```python
from build123d import *

# Parameters (mm, degrees)
SKETCH1_W           = 76.2
SKETCH1_H           = 76.2
SKETCH1_W_2         = 69.85
SKETCH1_H_2         = 69.85
EXTRUDE_THIN1_DEPTH = 38.1
SKETCH2_R           = 2.4892
CUT_EXTRUDE1_DEPTH  = 77.2


with BuildPart() as part:
    # Sketch1 → Extrude-Thin1 (new body, symmetric)
    with BuildSketch(Plane.XY):
        Rectangle(SKETCH1_W, SKETCH1_H)
        Rectangle(SKETCH1_W_2, SKETCH1_H_2, mode=Mode.SUBTRACT)
    extrude(amount=EXTRUDE_THIN1_DEPTH, both=True)

    # Sketch2 → Cut-Extrude1 (cut, through all)
    with BuildSketch(Plane.XZ.offset(38.1)):
        with Locations((0, 12.7)):
            Circle(SKETCH2_R)
        with Locations((0, -12.7)):
            Circle(SKETCH2_R)
    extrude(amount=-CUT_EXTRUDE1_DEPTH, mode=Mode.SUBTRACT)


solid = part.part
```
Here's how the part is built. I have some questions about the finished solid (model axes, mm). A direction names the side the tool comes from. Give positions to 0.01 mm unless a question says otherwise; leave off trailing zeros. Write each loop counter-clockwise with the first axis right and the second up, starting at its lowest first coordinate (ties: lowest second). Pieces come first, ordered by that corner, then holes. Notation, with made-up numbers: (62, -8) -> (107, -8) arc R25 cw to (107, 4) -> close; hole circle Ø6 at (4.5, 39). An arc over 180 degrees is marked (long way). Use one line per item in the form item = value.
1) I'm going to push a flat-ended pin straight in: pin 1 (4 mm diameter, centred on x = 0, z = 12.7, fed in from -Y). Where does the tip first touch, or does it pass through?
Verdict:
pin_1 = through
2) If I drill on L1, parallel to X at y = 20, z = -30.5 (3 decimals); L2, parallel to Z at x = 0, y = 35.7, over which ranges is the centre line in solid material (lowest first)? Write a range as [from, to].
Verdict:
L1 = [-38.1, -34.925], [34.925, 38.1]
L2 = [-38.1, -15.19], [-10.21, 10.21], [15.19, 38.1]
3) On a 3-axis mill with a long thin cutter (end or side, diameter ignored), from which of +Z, -Z, +X, -X, +Y, -Y can I reach the whole of each face in a straight line? I mean faces 4 (the face through (-3, -37, 38.1)), 5 (the face through (34.925, 0, 1)). Say none if no direction works.
Verdict:
face_4 = +Z, +X, -X, +Y, -Y
face_5 = +Z, -Z
4) Suppose I cut it at B-B (y = 20). Please give me the cut outline in (x, z) (3 decimals), and give its area (3 significant figures).
Verdict:
outline = (-38.1, -38.1) -> (-34.925, -38.1) -> (-34.925, 38.1) -> (-38.1, 38.1) -> close; (34.925, -38.1) -> (38.1, -38.1) -> (38.1, 38.1) -> (34.925, 38.1) -> close
area = 484 mm2
5) Suppose I cut it at D-D (x = 0). Please give me the cut outline in (y, z) (3 decimals), and give its area (3 significant figures).
Verdict:
outline = (-38.1, -38.1) -> (-34.925, -38.1) -> (-34.925, -15.189) -> (-38.1, -15.189) -> close; (-38.1, -10.211) -> (-34.925, -10.211) -> (-34.925, 10.211) -> (-38.1, 10.211) -> close; (-38.1, 15.189) -> (-34.925, 15.189) -> (-34.925, 38.1) -> (-38.1, 38.1) -> close; (34.925, -38.1) -> (38.1, -38.1) -> (38.1, -15.189) -> (34.925, -15.189) -> close; (34.925, -10.211) -> (38.1, -10.211) -> (38.1, 10.211) -> (34.925, 10.211) -> close; (34.925, 15.189) -> (38.1, 15.189) -> (38.1, 38.1) -> (34.925, 38.1) -> close
area = 421 mm2
6) Suppose I cut it at A-A (z = 12.7). Please give me the cut outline in (x, y) (3 decimals), and give its area (3 significant figures).
Verdict:
outline = (-38.1, -38.1) -> (-2.489, -38.1) -> (-2.489, -34.925) -> (-34.925, -34.925) -> (-34.925, 34.925) -> (-2.489, 34.925) -> (-2.489, 38.1) -> (-38.1, 38.1) -> close; (2.489, -38.1) -> (38.1, -38.1) -> (38.1, 38.1) -> (2.489, 38.1) -> (2.489, 34.925) -> (34.925, 34.925) -> (34.925, -34.925) -> (2.489, -34.925) -> close
area = 896 mm2
7) We'd pull the mould along X, two halves only. Please class faces 1 (the face through (38.1, -1, 1)), 2 (the face through (0, -34.925, 1)), 3 (the face through (-38.1, -1, 1)): +X half, -X half, draft (parallel to the pull), parting line (faces both ways), or undercut.
Verdict:
face_1 = +X half
face_2 = undercut
face_3 = -X half
